Geometry: final body of the model. Coordinates: model frame, mm. Face numbers are marked on the shaded views. Round coordinates to 2 decimals unless told otherwise and drop trailing zeros. Write each loop counter-clockwise with the first axis right and the second up, starting at its lowest first coordinate (ties: lowest second). Pieces come first, ordered by that corner, then holes.
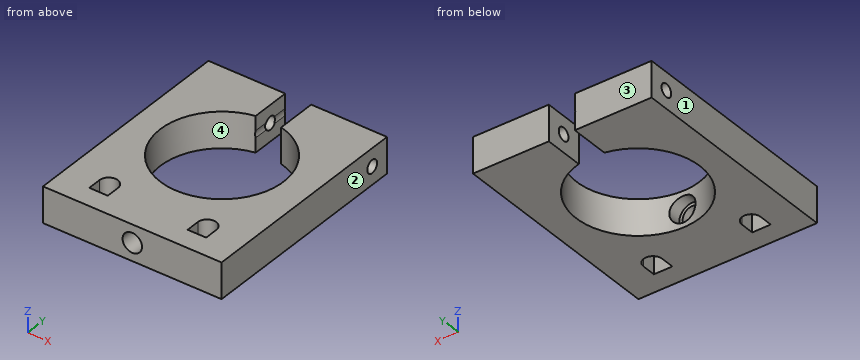
from build123d import *

# Parameters (mm, degrees)
SKETCH1_W           = 55
SKETCH1_H           = 18
BOSS_EXTRUDE1_DEPTH = 15
SKETCH2_W           = 55
SKETCH2_H           = 15
BOSS_EXTRUDE2_DEPTH = 50
SKETCH14_R          = 19
CUT_EXTRUDE14_DEPTH = 21
SKETCH6_W           = 8
SKETCH6_H           = 27.884489578
CUT_EXTRUDE3_DEPTH  = 50
SKETCH9_R           = 2
CUT_EXTRUDE5_DEPTH  = 55
CUT_EXTRUDE6_DEPTH  = 55
SKETCH16_W          = 55
SKETCH16_H          = 4
CUT_EXTRUDE16_DEPTH = 73
SKETCH17_R          = 3
CUT_EXTRUDE17_DEPTH = 89
SKETCH18_R          = 4
CUT_EXTRUDE18_DEPTH = 89


with BuildPart() as part:
    # Sketch1 → Boss-Extrude1 (new body)
    with BuildSketch(Plane.XY):
        with Locations((-27.5, 32.973684211)):
            Rectangle(SKETCH1_W, SKETCH1_H)
    extrude(amount=BOSS_EXTRUDE1_DEPTH)

    # Sketch2 → Boss-Extrude2 (add)
    with BuildSketch(Plane(origin=(0, 41.973684211, 0), x_dir=(1, 0, 0), z_dir=(0, 1, 0))):
        with Locations((-27.5, -7.5)):
            Rectangle(SKETCH2_W, SKETCH2_H)
    extrude(amount=BOSS_EXTRUDE2_DEPTH)

    # Sketch14 → Cut-Extrude14 (cut)
    with BuildSketch(Plane.XY.offset(15)):
        with Locations((-27.746201243, 61.173684211)):
            Circle(SKETCH14_R)
    extrude(amount=-CUT_EXTRUDE14_DEPTH, mode=Mode.SUBTRACT)

    # Sketch6 → Cut-Extrude3 (cut)
    with BuildSketch(Plane.XY.offset(15)):
        with Locations((-27.350353451, 79.894224222)):
            Rectangle(SKETCH6_W, SKETCH6_H)
    extrude(amount=-CUT_EXTRUDE3_DEPTH, mode=Mode.SUBTRACT)

    # Sketch9 → Cut-Extrude5 (cut)
    with BuildSketch(Plane.ZY.offset(55)):
        with Locations(Location((5.5, 85.888652512, 0), (0, 0, 270))):
            Circle(SKETCH9_R)
    extrude(amount=-CUT_EXTRUDE5_DEPTH, mode=Mode.SUBTRACT)

    # Sketch10 → Cut-Extrude6 (cut)
    with BuildSketch(Plane.XY.offset(15)):
        with BuildLine():
            Line((-9.5, 30.311825803), (-9.5, 34.473684211))
            ThreePointArc((-9.5, 34.473684211), (-12.35, 37.323684211), (-15.2, 34.473684211))
            Line((-15.2, 34.473684211), (-15.2, 30.311825803))
            Line((-15.2, 30.311825803), (-9.5, 30.311825803))
        make_face()
        with BuildLine():
            Line((-45.5, 30.311825803), (-39.8, 30.311825803))
            Line((-39.8, 30.311825803), (-39.8, 34.473684211))
            ThreePointArc((-39.8, 34.473684211), (-42.65, 37.323684211), (-45.5, 34.473684211))
            Line((-45.5, 34.473684211), (-45.5, 30.311825803))
        make_face()
    extrude(amount=-CUT_EXTRUDE6_DEPTH, mode=Mode.SUBTRACT)

    # Sketch16 → Cut-Extrude16 (cut)
    with BuildSketch(Plane(origin=(0, 23.973684211, 0), x_dir=(-1, 0, 0), z_dir=(0, -1, 0))):
        with Locations((27.5, -13)):
            Rectangle(SKETCH16_W, SKETCH16_H)
    extrude(amount=-CUT_EXTRUDE16_DEPTH, mode=Mode.SUBTRACT)

    # Sketch17 → Cut-Extrude17 (cut)
    with BuildSketch(Plane(origin=(0, 23.973684211, 0), x_dir=(-1, 0, 0), z_dir=(0, -1, 0))):
        with Locations(Location((27.5, -5.5, 0), (0, 0, 90))):
            Circle(SKETCH17_R)
    extrude(amount=-CUT_EXTRUDE17_DEPTH, mode=Mode.SUBTRACT)

    # Sketch18 → Cut-Extrude18 (cut)
    with BuildSketch(Plane(origin=(0, 38.5, 0), x_dir=(1, 0, 0), z_dir=(0, 1, 0))):
        with Locations(Location((-27.5, -5.5, 0), (0, 0, 90))):
            Circle(SKETCH18_R)
    extrude(amount=CUT_EXTRUDE18_DEPTH, mode=Mode.SUBTRACT)


solid = part.part
1) Section C-C on x = -27.5. Output: boundary loops of the cut face in (y, z), plus the area to 3 significant figures.
2) Section A-A on x = -11.5. Output: boundary loops of the cut face in (y, z), plus the area to 3 significant figures.
3) Draft query along X for the marked faces 1, 2, 3 and 4. Return one class per face: pulls with the +X half, pulls with the -X half, needs draft (parallel to the pull), parting line crosses it, or undercut.
4) First-contact query: P1, Ø2, axis at y = 55, z = 6, coming from the +X side; P2, Ø23, axis at x = -27.75, y = 61.17, coming from the -Z side; P3, Ø4, axis at x = -28, z = 4.5, coming from the +Y side. Flat tips, straight axial feed; report the tip coordinate or a pass-through.
5) Line query: probe 1 along X at (y, z) = (31, 5.5); probe 2 along X at (y, z) = (28, 5.5); probe 3 along Y at (x, z) = (-44.5, 3). Output: solid intervals per line, ascending.
6) Section D-D on y = 60. Output: boundary loops of the cut face in (x, z).
7) Section B-B on z = 5.5. State how many separate pieces and enclosed holes the cut face has, plus the area to 3 significant figures.
Filled in:
1. outline: (23.97, 0) - (42.18, 0) - (42.18, 1.5) - (38.5, 1.5) - (38.5, 2.5) - (23.97, 2.5) - close; (23.97, 8.5) - (38.5, 8.5) - (38.5, 9.5) - (42.18, 9.5) - (42.18, 11) - (23.97, 11) - close
1. area: 83.7 mm2
2. outline: (23.97, 0) - (30.31, 0) - (30.31, 11) - (23.97, 11) - close; (37.19, 0) - (51.32, 0) - (51.32, 11) - (37.19, 11) - close; (71.03, 0) - (91.97, 0) - (91.97, 11) - (71.03, 11) - close; hole circle Ø4 at (85.89, 5.5)
2. area: 443 mm2
3. face 1: pulls with the -X half
3. face 2: pulls with the +X half
3. face 3: needs draft
3. face 4: undercut
4. P1: stops at x = 0
4. P2: passes through
4. P3: stops at y = 38.5
5. probe 1: x = -55 to -45.5, -39.8 to -30.5, -24.5 to -15.2, -9.5 to 0
5. probe 2: x = -55 to -30.5, -24.5 to 0
5. probe 3: y = 23.97 to 30.31, 36.64 to 52.21, 70.14 to 91.97
6. outline: (-55, 0) - (-46.71, 0) - (-46.71, 11) - (-55, 11) - close; (-8.78, 0) - (0, 0) - (0, 11) - (-8.78, 11) - close
7. separate pieces: 4
7. enclosed holes: 2
7. area: 2,130 mm2
